```python
from build123d import *
from OCP.BRepFilletAPI import BRepFilletAPI_MakeChamfer

# Parameters (mm, degrees)
SKETCH1_R           = 9
BOSS_EXTRUDE1_DEPTH = 12
SKETCH1_3_R         = 1.95
BOSS_EXTRUDE2_DEPTH = 2
BOSS_EXTRUDE3_START = -5
SKETCH4_R           = 11.5
SKETCH4_R_2         = 9
BOSS_EXTRUDE3_DEPTH = 5
CUT_EXTRUDE2_DEPTH  = 3
CHAMFER1_SIZE       = 0.8
CHAMFER1_SIZE2      = 0.671279705


with BuildPart() as part:
    # Sketch1 → Boss-Extrude1 (new body)
    with BuildSketch(Plane(origin=(0, 0, 0), x_dir=(1, 0, 0), z_dir=(0, 1, 0))):
        with Locations(Location((0, 0, 0), (0, 0, 270))):
            Circle(SKETCH1_R)
    extrude(amount=BOSS_EXTRUDE1_DEPTH)

    # Sketch1_3 → Boss-Extrude2 (add)
    with BuildSketch(Plane(origin=(0, 0, 0), x_dir=(1, 0, 0), z_dir=(0, 1, 0))):
        with Locations(Location((-6, 0, 0), (0, 0, 270))):
            Circle(SKETCH1_3_R)
        with Locations(Location((0, 6, 0), (0, 0, 270))):
            Circle(SKETCH1_3_R)
        with Locations(Location((6, 0, 0), (0, 0, 270))):
            Circle(SKETCH1_3_R)
        with Locations(Location((0, -6, 0), (0, 0, 270))):
            Circle(SKETCH1_3_R)
    extrude(amount=-BOSS_EXTRUDE2_DEPTH)

    # Sketch4 → Boss-Extrude3 (add)
    with BuildSketch(Plane(origin=(0, 12, 0), x_dir=(1, 0, 0), z_dir=(0, 1, 0)).offset(BOSS_EXTRUDE3_START)):
        with Locations(Location((0, 0, 0), (0, 0, 270))):
            Circle(SKETCH4_R)
        with Locations(Location((0, 0, 0), (0, 0, 270))):
            Circle(SKETCH4_R_2, mode=Mode.SUBTRACT)
    extrude(amount=BOSS_EXTRUDE3_DEPTH)

    # Sketch3 → Cut-Extrude2 (cut)
    with BuildSketch(Plane(origin=(0, 12, 0), x_dir=(1, 0, 0), z_dir=(0, 1, 0))):
        with BuildLine():
            Line((1.65, 12.188826851), (1.65, 3.983452378))
            Line((1.65, 3.983452378), (7.452075932, 9.78552831))
            ThreePointArc((7.452075932, 9.78552831), (8.697413409, 8.697413409), (9.78552831, 7.452075932))
            Line((9.78552831, 7.452075932), (3.983452378, 1.65))
            Line((3.983452378, 1.65), (12.188826851, 1.65))
            ThreePointArc((12.188826851, 1.65), (12.3, 0), (12.188826851, -1.65))
            Line((12.188826851, -1.65), (3.983452378, -1.65))
            Line((3.983452378, -1.65), (9.78552831, -7.452075932))
            ThreePointArc((9.78552831, -7.452075932), (8.697413409, -8.697413409), (7.452075932, -9.78552831))
            Line((7.452075932, -9.78552831), (1.65, -3.983452378))
            Line((1.65, -3.983452378), (1.65, -12.188826851))
            ThreePointArc((1.65, -12.188826851), (0, -12.3), (-1.65, -12.188826851))
            Line((-1.65, -12.188826851), (-1.65, -3.983452378))
            Line((-1.65, -3.983452378), (-7.452075932, -9.78552831))
            ThreePointArc((-7.452075932, -9.78552831), (-8.697413409, -8.697413409), (-9.78552831, -7.452075932))
            Line((-9.78552831, -7.452075932), (-3.983452378, -1.65))
            Line((-3.983452378, -1.65), (-12.188826851, -1.65))
            ThreePointArc((-12.188826851, -1.65), (-12.3, 0), (-12.188826851, 1.65))
            Line((-12.188826851, 1.65), (-3.983452378, 1.65))
            Line((-3.983452378, 1.65), (-9.78552831, 7.452075932))
            ThreePointArc((-9.78552831, 7.452075932), (-8.697413409, 8.697413409), (-7.452075932, 9.78552831))
            Line((-7.452075932, 9.78552831), (-1.65, 3.983452378))
            Line((-1.65, 3.983452378), (-1.65, 12.188826851))
            ThreePointArc((-1.65, 12.188826851), (0, 12.3), (1.65, 12.188826851))
        make_face()
    extrude(amount=-CUT_EXTRUDE2_DEPTH, mode=Mode.SUBTRACT)

    # Chamfer1: one chamfer whose edges measure the first distance from different faces: ONE call of the kernel's chamfer builder (chamfer() names one face for all edges)
    chamfer1_edges_1 = [part.edges().sort_by_distance(p)[0] for p in [
        (-7.682233636, 12, -1.65),
    ]]
    chamfer1_side_1 = [part.faces().sort_by_distance(p)[0] for p in [
        (-7.682233636, 10.5, -1.65),
    ]]
    chamfer1_edges_2 = [part.edges().sort_by_distance(p)[0] for p in [
        (-6.598885687, 12, 4.265433309),
    ]]
    chamfer1_side_2 = [part.faces().sort_by_distance(p)[0] for p in [
        (-6.598885687, 10.5, 4.265433309),
    ]]
    chamfer1_edges_3 = [part.edges().sort_by_distance(p)[0] for p in [
        (-1.65, 12, 7.682233636),
    ]]
    chamfer1_side_3 = [part.faces().sort_by_distance(p)[0] for p in [
        (-1.65, 10.5, 7.682233636),
    ]]
    chamfer1_edges_4 = [part.edges().sort_by_distance(p)[0] for p in [
        (4.265433309, 12, 6.598885687),
    ]]
    chamfer1_side_4 = [part.faces().sort_by_distance(p)[0] for p in [
        (4.265433309, 10.5, 6.598885687),
    ]]
    chamfer1_edges_5 = [part.edges().sort_by_distance(p)[0] for p in [
        (7.682233636, 12, 1.65),
    ]]
    chamfer1_side_5 = [part.faces().sort_by_distance(p)[0] for p in [
        (7.682233636, 10.5, 1.65),
    ]]
    chamfer1_edges_6 = [part.edges().sort_by_distance(p)[0] for p in [
        (6.598885687, 12, -4.265433309),
    ]]
    chamfer1_side_6 = [part.faces().sort_by_distance(p)[0] for p in [
        (6.598885687, 10.5, -4.265433309),
    ]]
    chamfer1_edges_7 = [part.edges().sort_by_distance(p)[0] for p in [
        (1.65, 12, -7.682233636),
    ]]
    chamfer1_side_7 = [part.faces().sort_by_distance(p)[0] for p in [
        (1.65, 10.5, -7.682233636),
    ]]
    chamfer1_edges_8 = [part.edges().sort_by_distance(p)[0] for p in [
        (-4.265433309, 12, -6.598885687),
    ]]
    chamfer1_side_8 = [part.faces().sort_by_distance(p)[0] for p in [
        (-4.265433309, 10.5, -6.598885687),
    ]]
    chamfer1_edges_9 = [part.edges().sort_by_distance(p)[0] for p in [
        (-6.598885687, 12, -4.265433309),
    ]]
    chamfer1_side_9 = [part.faces().sort_by_distance(p)[0] for p in [
        (-6.598885687, 10.5, -4.265433309),
    ]]
    chamfer1_edges_10 = [part.edges().sort_by_distance(p)[0] for p in [
        (-1.65, 12, -7.682233636),
    ]]
    chamfer1_side_10 = [part.faces().sort_by_distance(p)[0] for p in [
        (-1.65, 10.5, -7.682233636),
    ]]
    chamfer1_edges_11 = [part.edges().sort_by_distance(p)[0] for p in [
        (4.265433309, 12, -6.598885687),
    ]]
    chamfer1_side_11 = [part.faces().sort_by_distance(p)[0] for p in [
        (4.265433309, 10.5, -6.598885687),
    ]]
    chamfer1_edges_12 = [part.edges().sort_by_distance(p)[0] for p in [
        (7.682233636, 12, -1.65),
    ]]
    chamfer1_side_12 = [part.faces().sort_by_distance(p)[0] for p in [
        (7.682233636, 10.5, -1.65),
    ]]
    chamfer1_edges_13 = [part.edges().sort_by_distance(p)[0] for p in [
        (6.598885687, 12, 4.265433309),
    ]]
    chamfer1_side_13 = [part.faces().sort_by_distance(p)[0] for p in [
        (6.598885687, 10.5, 4.265433309),
    ]]
    chamfer1_edges_14 = [part.edges().sort_by_distance(p)[0] for p in [
        (-4.265433309, 12, 6.598885687),
    ]]
    chamfer1_side_14 = [part.faces().sort_by_distance(p)[0] for p in [
        (-4.265433309, 10.5, 6.598885687),
    ]]
    chamfer1_edges_15 = [part.edges().sort_by_distance(p)[0] for p in [
        (-7.682233636, 12, 1.65),
    ]]
    chamfer1_side_15 = [part.faces().sort_by_distance(p)[0] for p in [
        (-7.682233636, 10.5, 1.65),
    ]]
    chamfer1 = BRepFilletAPI_MakeChamfer(part.part.solid().wrapped)
    for e in chamfer1_edges_1:
        chamfer1.Add(CHAMFER1_SIZE, CHAMFER1_SIZE2, e.wrapped, chamfer1_side_1[0].wrapped)  # the first distance lies on this face
    for e in chamfer1_edges_2:
        chamfer1.Add(CHAMFER1_SIZE, CHAMFER1_SIZE2, e.wrapped, chamfer1_side_2[0].wrapped)  # the first distance lies on this face
    for e in chamfer1_edges_3:
        chamfer1.Add(CHAMFER1_SIZE, CHAMFER1_SIZE2, e.wrapped, chamfer1_side_3[0].wrapped)  # the first distance lies on this face
    for e in chamfer1_edges_4:
        chamfer1.Add(CHAMFER1_SIZE, CHAMFER1_SIZE2, e.wrapped, chamfer1_side_4[0].wrapped)  # the first distance lies on this face
    for e in chamfer1_edges_5:
        chamfer1.Add(CHAMFER1_SIZE, CHAMFER1_SIZE2, e.wrapped, chamfer1_side_5[0].wrapped)  # the first distance lies on this face
    for e in chamfer1_edges_6:
        chamfer1.Add(CHAMFER1_SIZE, CHAMFER1_SIZE2, e.wrapped, chamfer1_side_6[0].wrapped)  # the first distance lies on this face
    for e in chamfer1_edges_7:
        chamfer1.Add(CHAMFER1_SIZE, CHAMFER1_SIZE2, e.wrapped, chamfer1_side_7[0].wrapped)  # the first distance lies on this face
    for e in chamfer1_edges_8:
        chamfer1.Add(CHAMFER1_SIZE, CHAMFER1_SIZE2, e.wrapped, chamfer1_side_8[0].wrapped)  # the first distance lies on this face
    for e in chamfer1_edges_9:
        chamfer1.Add(CHAMFER1_SIZE, CHAMFER1_SIZE2, e.wrapped, chamfer1_side_9[0].wrapped)  # the first distance lies on this face
    for e in chamfer1_edges_10:
        chamfer1.Add(CHAMFER1_SIZE, CHAMFER1_SIZE2, e.wrapped, chamfer1_side_10[0].wrapped)  # the first distance lies on this face
    for e in chamfer1_edges_11:
        chamfer1.Add(CHAMFER1_SIZE, CHAMFER1_SIZE2, e.wrapped, chamfer1_side_11[0].wrapped)  # the first distance lies on this face
    for e in chamfer1_edges_12:
        chamfer1.Add(CHAMFER1_SIZE, CHAMFER1_SIZE2, e.wrapped, chamfer1_side_12[0].wrapped)  # the first distance lies on this face
    for e in chamfer1_edges_13:
        chamfer1.Add(CHAMFER1_SIZE, CHAMFER1_SIZE2, e.wrapped, chamfer1_side_13[0].wrapped)  # the first distance lies on this face
    for e in chamfer1_edges_14:
        chamfer1.Add(CHAMFER1_SIZE, CHAMFER1_SIZE2, e.wrapped, chamfer1_side_14[0].wrapped)  # the first distance lies on this face
    for e in chamfer1_edges_15:
        chamfer1.Add(CHAMFER1_SIZE, CHAMFER1_SIZE2, e.wrapped, chamfer1_side_15[0].wrapped)  # the first distance lies on this face
    add(Compound.cast(chamfer1.Shape()), mode=Mode.REPLACE)


solid = part.part
```
Read the model definition and answer for the solid it produces. Units are mm, in the model's axes. A direction names the side the tool comes from. Coordinates: 2 decimals unless noted, no trailing zeros. Loops run counter-clockwise (first coordinate to the right, second up) from the corner with the lowest first, then second, coordinate; pieces in that order, holes last. Notation, with made-up numbers: (75.5, 74) - (101.5, 74) arc R19 ccw to (101.5, 83) - close; hole circle Ø1 at (20, 67). An arc over 180 degrees is marked (long way). Answer in a Markdown table with one row per item.
1. Given pin 1 (5 mm diameter, centred on x = -6.5, y = 6, fed in from -Z); pin 2 (2.5 mm diameter, centred on x = 6.5, y = 10.5, fed in from +Z); pin 3 (3 mm diameter, centred on x = 7.5, y = 7, fed in from -Z), each flat-ended and moving along its own axis, determine where each tip first touches the part or whether it passes through.
Conclusion:
| item | result |
|---|---|
| pin 1 | stops at z = -10.7 |
| pin 2 | stops at z = 10.23 |
| pin 3 | stops at z = -9.81 |
2. Determine the mould class of faces 1 (the face through (9, 12, 4)), 2 (the face through (-4.405, 8.909, 10.623)), 3 (the face through (4.569, 11.606, -7.384)) for opening direction Z: +Z half, -Z half, draft (parallel to the pull), parting line (faces both ways), or undercut.
Conclusion:
| item | result |
|---|---|
| face 1 | draft |
| face 2 | parting line |
| face 3 | undercut |
3. Straight lines are drawn through the part: line 1 (Z direction, x = -5.75, y = 11); line 2 (X direction, y = 10.75, z = 6.75); line 3 (Y direction, x = -10, z = -3.5). For each, find the intervals that lie inside material, in ascending order.
Conclusion:
| item | result |
|---|---|
| line 1 | z = -9.96 to -8.08, -3.42 to -1.65, 1.65 to 3.42, 8.08 to 9.96 |
| line 2 | x = -9.31 to -9.08, -4.42 to -1.65, 1.65 to 4.42, 9.08 to 9.31 |
| line 3 | y = 7 to 12 |
4. Find section A-A, the plane y = 10.5. Write down the section's boundary in (x, z), then the cut area to 3 significant figures.
Conclusion:
| item | result |
|---|---|
| outline | (-11.38, -1.65) arc R11.5 ccw to (-9.21, -6.88) - (-3.98, -1.65) - close; (-11.38, 1.65) - (-3.98, 1.65) - (-9.21, 6.88) arc R11.5 ccw to start; (-6.88, -9.21) arc R11.5 ccw to (-1.65, -11.38) - (-1.65, -3.98) - close; (-6.88, 9.21) - (-1.65, 3.98) - (-1.65, 11.38) arc R11.5 ccw to start; (1.65, -11.38) arc R11.5 ccw to (6.88, -9.21) - (1.65, -3.98) - close; (1.65, 3.98) - (6.88, 9.21) arc R11.5 ccw to (1.65, 11.38) - close; (3.98, -1.65) - (9.21, -6.88) arc R11.5 ccw to (11.38, -1.65) - close; (3.98, 1.65) - (11.38, 1.65) arc R11.5 ccw to (9.21, 6.88) - close |
| area | 166 mm² |
5. Which of the six approach directions +Z, -Z, +X, -X, +Y, -Y give full straight-line access (tool end or side, diameter ignored) to faces 4 (the face through (-4.06, 11.61, -6.88)), 5 (the face through (8, 10, -1.65)), 6 (the face through (1.65, 11, 8))?
Conclusion:
| item | result |
|---|---|
| face 4 | +Y |
| face 5 | +X, -X, +Y |
| face 6 | +Z, -Z, +Y |
6. Find section C-C, the plane y = -0.5. Write down the section's boundary in (x, z), then the cut area to 3 significant figures.
Conclusion:
| item | result |
|---|---|
| outline | circle Ø3.9 at (-6, 0); circle Ø3.9 at (0, -6); circle Ø3.9 at (0, 6); circle Ø3.9 at (6, 0) |
| area | 47.8 mm² |
7. Find section B-B, the plane x = 0. Write down the section's boundary in (y, z).
Conclusion:
| item | result |
|---|---|
| outline | (-2, -7.95) - (0, -7.95) - (0, -9) - (7, -9) - (7, -11.5) - (9, -11.5) - (9, 11.5) - (7, 11.5) - (7, 9) - (0, 9) - (0, 7.95) - (-2, 7.95) - (-2, 4.05) - (0, 4.05) - (0, -4.05) - (-2, -4.05) - close |
